from build123d import *

# Parameters (mm, degrees)
SKETCH_1_R               = 25
SKETCH_1_R_2             = 1.25
EXTRUDE_1_DEPTH          = 3
SKETCH_3_R               = 10.5
SKETCH_3_R_2             = 4
SKETCH_3_R_3             = 1
CUT_EXTRUDE_1_DEPTH      = 1
CUT_EXTRUDE_2_DEPTH      = 36.482389998
CUT_EXTRUDE_2_DEPTH_BACK = 36.482389998
SKETCH_3_2_R             = 1
SKETCH_3_2_R_2           = 4
CUT_EXTRUDE_5_DEPTH      = 10
FILLET_2_R               = 5
FILLET_3_R               = 10


with BuildPart() as part:
    # Sketch 1 → Extrude 1 (new body)
    with BuildSketch(Plane.XY):
        Circle(SKETCH_1_R)
        with Locations((0, 22)):
            Circle(SKETCH_1_R_2, mode=Mode.SUBTRACT)
        with Locations((22, 0)):
            Circle(SKETCH_1_R_2, mode=Mode.SUBTRACT)
        with Locations((0, -22)):
            Circle(SKETCH_1_R_2, mode=Mode.SUBTRACT)
    extrude(amount=EXTRUDE_1_DEPTH)

    # Sketch 3 → Cut-Extrude 1 (cut)
    with BuildSketch(Plane(origin=(0, 0, 0), x_dir=(-1, 0, 0), z_dir=(0, 0, -1))):
        Circle(SKETCH_3_R)
        Circle(SKETCH_3_R_2, mode=Mode.SUBTRACT)
        with Locations((0, 6.2)):
            Circle(SKETCH_3_R_3, mode=Mode.SUBTRACT)
        with Locations((0, -6.2)):
            Circle(SKETCH_3_R_3, mode=Mode.SUBTRACT)
    extrude(amount=-CUT_EXTRUDE_1_DEPTH, mode=Mode.SUBTRACT)

    # Sketch 3_2 → Cut-Extrude 2 (cut, two sides: drawn at the far end of the back side and taken through both)
    with BuildSketch(Plane(origin=(0, 0, 0), x_dir=(-1, 0, 0), z_dir=(0, 0, -1)).offset(-CUT_EXTRUDE_2_DEPTH_BACK)):
        with Locations((0, 6.2)):
            Circle(SKETCH_3_2_R)
        Circle(SKETCH_3_2_R_2)
        with Locations((0, -6.2)):
            Circle(SKETCH_3_2_R)
    extrude(amount=CUT_EXTRUDE_2_DEPTH + CUT_EXTRUDE_2_DEPTH_BACK, mode=Mode.SUBTRACT)

    # Sketch 5 → Cut-Extrude 5 (cut)
    with BuildSketch(Plane(origin=(0, 0, 0), x_dir=(-1, 0, 0), z_dir=(0, 0, -1))):
        with BuildLine():
            Line((-24.613742187, 4.377635842), (-8.838834765, 8.838834765))
            Line((-8.838834765, 8.838834765), (-4.377635842, 24.613742187))
            ThreePointArc((-4.377635842, 24.613742187), (-17.67766953, 17.67766953), (-24.613742187, 4.377635842))
        make_face()
        with BuildLine():
            Line((-4.377635842, -24.613742187), (-8.838834765, -8.838834765))
            Line((-8.838834765, -8.838834765), (-24.613742187, -4.377635842))
            ThreePointArc((-24.613742187, -4.377635842), (-17.67766953, -17.67766953), (-4.377635842, -24.613742187))
        make_face()
        with BuildLine():
            Line((9, -16.733200531), (9, -23.323807579))
            ThreePointArc((9, -23.323807579), (25, 0), (9, 23.323807579))
            Line((9, 23.323807579), (9, 16.733200531))
            ThreePointArc((9, 16.733200531), (19, 0), (9, -16.733200531))
        make_face()
    extrude(amount=-CUT_EXTRUDE_5_DEPTH, mode=Mode.SUBTRACT)

    # Fillet 2
    fillet_2_edges = [part.edges().sort_by_distance(p)[0] for p in [
        (24.613742187, 4.377635842, 1.5),
        (4.377635842, 24.613742187, 1.5),
        (4.377635842, -24.613742187, 1.5),
        (24.613742187, -4.377635842, 1.5),
        (-9, 23.323807579, 1.5),
        (-9, -23.323807579, 1.5),
    ]]
    fillet(fillet_2_edges, radius=FILLET_2_R)

    # Fillet 3
    fillet_3_edges = [part.edges().sort_by_distance(p)[0] for p in [
        (8.838834765, 8.838834765, 1.5),
        (8.838834765, -8.838834765, 1.5),
        (-9, -16.733200531, 1.5),
        (-9, 16.733200531, 1.5),
    ]]
    fillet(fillet_3_edges, radius=FILLET_3_R)


solid = part.part
Here's how the part is built. I have some questions about the finished solid (model axes, mm). Coordinates: 2 decimals unless noted, no trailing zeros. Loops run counter-clockwise (first coordinate to the right, second up) from the corner with the lowest first, then second, coordinate; pieces in that order, holes last. Notation, with made-up numbers: (0.5, -31.5) -> (4.5, -31.5) arc R25 ccw to (4.5, 7.5) -> close; hole circle Ø4 at (-10, 47). An arc over 180 degrees is marked (long way). Use one line per item in the form item = value. Start each with the question number.
(1) We'd pull the mould along Y, two halves only. Please class faces 1 (the face through (9.92, 9.82, 1.52)), 2 (the face through (0.867, -3.905, 2.014)), 3 (the face through (-19, 0, 1)): pulls with the +Y half, pulls with the -Y half, needs draft (parallel to the pull), parting line crosses it, or undercut.
(2) If we section it at D-D (z = 2.35): Give the number of separate pieces and of enclosed holes in the cut face, then the cut area to 3 significant figures.
(3) If we section it at A-A (x = 0): Please give me the cut outline in (y, z), then the cut area to 3 significant figures.
(4) If we section it at B-B (y = 0): Please give me the cut outline in (x, z), then the cut area to 3 significant figures.
(5) If we section it at C-C (y = -6.2): Please give me the cut outline in (x, z).
(6) Will these pins go through, and if not, where does the flat tip stop? pin 1 (1 mm diameter, centred on x = 2.5, z = 1, fed in from +Y); pin 2 (6.5 mm diameter, centred on x = 4.5, y = 4.5, fed in from -Z); pin 3 (7 mm diameter, centred on x = 0, y = 0, fed in from -Z); pin 4 (1 mm diameter, centred on y = -7.5, z = 1.5, fed in from -X).
(7) Please list where these lines run through material, in increasing order: line 1 along Y through (x, z) = (0, 0.25); line 2 along Y through (x, z) = (0, 2.4); line 3 along Y through (x, z) = (-1, 0.75).
Verdict:
q1.face_1 = pulls with the +Y half
q1.face_2 = undercut
q1.face_3 = parting line crosses it
q2.separate_pieces = 1
q2.enclosed_holes = 6
q2.area = 1,190 mm²
q3.outline = (-25, 0) -> (-23.25, 0) -> (-23.25, 3) -> (-25, 3) -> close; (-20.75, 0) -> (-10.5, 0) -> (-10.5, 1) -> (-7.2, 1) -> (-7.2, 3) -> (-20.75, 3) -> close; (-5.2, 1) -> (-4, 1) -> (-4, 3) -> (-5.2, 3) -> close; (4, 1) -> (5.2, 1) -> (5.2, 3) -> (4, 3) -> close; (7.2, 1) -> (10.5, 1) -> (10.5, 0) -> (20.75, 0) -> (20.75, 3) -> (7.2, 3) -> close; (23.25, 0) -> (25, 0) -> (25, 3) -> (23.25, 3) -> close
q3.area = 90.0 mm²
q4.outline = (-19, 0) -> (-10.5, 0) -> (-10.5, 1) -> (-4, 1) -> (-4, 3) -> (-19, 3) -> close; (4, 1) -> (10.5, 1) -> (10.5, 0) -> (20.75, 0) -> (20.75, 3) -> (4, 3) -> close; (23.25, 0) -> (25, 0) -> (25, 3) -> (23.25, 3) -> close
q4.area = 87.5 mm²
q5.outline = (-17.96, 0) -> (-8.47, 0) -> (-8.47, 1) -> (-1, 1) -> (-1, 3) -> (-17.96, 3) -> close; (1, 1) -> (8.47, 1) -> (8.47, 0) -> (18.17, 0) -> (18.17, 3) -> (1, 3) -> close
q6.pin_1 = 24.76
q6.pin_2 = 1
q6.pin_3 = through
q6.pin_4 = -17.66
q7.line_1 = -25 to -23.25, -20.75 to -10.5, 10.5 to 20.75, 23.25 to 25
q7.line_2 = -25 to -23.25, -20.75 to -7.2, -5.2 to -4, 4 to 5.2, 7.2 to 20.75, 23.25 to 25
q7.line_3 = -24.98 to -22.75, -21.25 to -10.45, 10.45 to 21.25, 22.75 to 24.98
